```python
from build123d import *

# Parameters (mm, degrees)
F0_R     = 10.95
F1_DEPTH = 3
F2_R     = 2.915
F3_DEPTH = 6.5


# Not quite as in the source:
# - a fillet or chamfer that OpenCascade refuses, or shapes differently, is made with other operations: its cross-section is extruded or revolved along the edge and cut away or added


with BuildPart() as f1:
    # F0 (on Front) → F1 (new body)
    with BuildSketch(Plane.XZ):
        Circle(F0_R)
    extrude(amount=F1_DEPTH)

    # F2 (on face) → F3 (join)
    with BuildSketch(Plane.XZ.offset(3)):
        Circle(F2_R)
    extrude(amount=F3_DEPTH)

    # F4: fillet of radius 3.81 on 1 edges, made by hand

    # F4_s1 → F4_t2 (revolve, cut)
    with BuildSketch(Plane.XY):
        with BuildLine():
            ThreePointArc((10.95, -3), (9.6177045238, -0.843335206), (7.2270979062, 0))
            Line((7.2270979062, 0), (10.95, 0))
            Line((10.95, 0), (10.95, -3))
        make_face()
    revolve(axis=Axis((0, 0, 0), (0, -1, 0)), mode=Mode.SUBTRACT)


solid = f1.part
```
The listing builds one solid part. Answer for the finished solid, in the listing's coordinates (mm). A direction names the side the tool comes from. Round coordinates to 2 decimals unless told otherwise and drop trailing zeros. Loops run counter-clockwise (first coordinate to the right, second up) from the corner with the lowest first, then second, coordinate; pieces in that order, holes last. Notation, with made-up numbers: (65, 86.5) -> (98, 86.5) arc R27 ccw to (98, 116.5) -> close; hole circle Ø6 at (75.25, -29). An arc over 180 degrees is marked (long way). Use one line per item in the form item = value.
1. The part is cut by section A-A on z = 0. Determine the outline of the cut face in (x, y) (3 decimals).
Answer key:
outline = (-10.95, -3) -> (-2.915, -3) -> (-2.915, -9.5) -> (2.915, -9.5) -> (2.915, -3) -> (10.95, -3) arc R3.81 ccw to (7.227, 0) -> (-7.227, 0) arc R3.81 ccw to start
2. Flat-ended cylindrical pins translate along their axes: pin 1 Ø2 at (x, z) = (-6.5, -6.5) entering from -Y; pin 2 Ø3 at (y, z) = (-5.5, 2.5) entering from +X; pin 3 Ø1 at (y, z) = (-8, -1) entering from +X. Find the tip coordinate at first contact, or state that the pin passes through.
Answer key:
pin_1 = -3
pin_2 = 2.74
pin_3 = 2.87
3. Find the intervals of material crossed by probe 1 along Y at (x, z) = (6, 1); probe 2 along Z at (x, y) = (2.25, -7.5); probe 3 along Z at (x, y) = (1.75, -7.75), in increasing order. Write a range as [from, to].
Answer key:
probe_1 = [-3, 0]
probe_2 = [-1.85, 1.85]
probe_3 = [-2.33, 2.33]
4. The part is cut by section B-B on x = 0. Determine the outline of the cut face in (y, z) (3 decimals).
Answer key:
outline = (-9.5, -2.915) -> (-3, -2.915) -> (-3, -10.95) arc R3.81 ccw to (0, -7.227) -> (0, 7.227) arc R3.81 ccw to (-3, 10.95) -> (-3, 2.915) -> (-9.5, 2.915) -> close
5. The part is cut by section C-C on y = -3.5. Determine the outline of the cut face in (x, z) (3 decimals), and give its area (3 significant figures).
Answer key:
outline = circle Ø5.83 at (0, 0)
area = 26.7 mm²
6. A tool of negligible diameter and unlimited length cuts with its end or side. For faces 1 (the flat face through (0, 0, 0)), 2 (the flat face through (2.3, -3, -2.3)), from which of +Z, -Z, +X, -X, +Y, -Y can it reach the whole face along a straight path? Write none if from no direction.
Answer key:
face_1 = +Z, -Z, +X, -X, +Y
face_2 = -Y
